Here's how the part is built. I have some questions about the finished solid (model axes, mm). A direction names the side the tool comes from. Round coordinates to 2 decimals unless told otherwise and drop trailing zeros. Loops run counter-clockwise (first coordinate to the right, second up) from the corner with the lowest first, then second, coordinate; pieces in that order, holes last. Notation, with made-up numbers: M 54,53.5 L 88,53.5 A25 ccw 88,80.5 Z; hole C -30,88.5 d11. An arc over 180 degrees is marked long. Answer as a JSON object with one key per item and string values.
Autodesk Inventor part; units mm, degrees
ref_plane "YZ Plane" through (0, 0, 0) normal (1, 0, 0) x (0, 1, 0)
ref_plane "XZ Plane" through (0, 0, 0) normal (0, 1, 0) x (-1, 0, 0)
ref_plane "XY Plane" through (0, 0, 0) normal (0, 0, 1) x (1, 0, 0)
sketch "Sketch1" plane through (0, 0, 0) normal (0, 0, 1) x (1, 0, 0)
  circle A0 centre (0, 0) radius 28 construction
  line L0 (75, -135) -> (-75, -135) construction
  line L1 (-75, -135) -> (-75, 65) construction
  line L2 (-75, 65) -> (75, 65) construction
  line L3 (75, 65) -> (75, -135) construction
  line L4 (75, -135) -> (-75, 65) construction
  line L5 (-75, -135) -> (75, 65) construction
  circle A1 centre (0, 0) radius 20
  circle A2 centre (-38.0423, -27.6393) radius 20
  circle A3 centre (-23.5114, -72.3607) radius 20
  circle A4 centre (23.5114, -72.3607) radius 20
  circle A5 centre (38.0423, -27.6393) radius 20
  circle A6 centre (0, -40) radius 62.5
  circle A7 centre (0, -40) radius 1.5
  circle A8 centre (0, -40) radius 4.05
  circle A9 centre (38.0423, -27.6393) radius 22.5 construction
  circle A10 centre (0, 0) radius 22.5 construction
  circle A11 centre (-38.0423, -27.6393) radius 22.5 construction
  circle A12 centre (-23.5114, -72.3607) radius 22.5 construction
  circle A13 centre (23.5114, -72.3607) radius 22.5 construction
  point P0 (0, -35)
  point P1 (0, -32)
  dimension "d0" = 56
  dimension "d1" = 150
  dimension "d2" = 200
  dimension "d3" = 135
  dimension "d4" = 40
  dimension "d7" = 360
  dimension "d9" = 40
  dimension "d10" = 125
  dimension "d11" = 3
  dimension "d12" = 8.1
  dimension "d17" = 45
  dimension "d20" = 360
  dimension "d22" = 8
extrude "Extrusion1" add sketch "Sketch1" along normal blind 10 contours A6
extrude "Extrusion2" add sketch "Sketch1" along normal blind 7 contours A8
hole "Hole1" at (0, -40, 0) at (0, -32, 0) direction (0, 0, 1) diameter 2 end through all
properties part number "FilterWheel-M40-5pos"
Item 1: For faces 1 (the face through (0, -42, 7)), 2 (the face through (20.91, -92.19, 4.93)), which set-ups out of +Z, -Z, +X, -X, +Y, -Y let a thin tool reach every point of the face, with its end or its side?
Solution:
{"face 1": "+Z", "face 2": "+Z, -Z"}
Item 2: If I drill on L1, parallel to Y at x = 0, z = 4.75; L2, parallel to Y at x = 0, z = 7.25; L3, parallel to Y at x = 36.5, z = 6.75, over which ranges is the centre line in solid material (lowest first)? Write a range as from..to.
Solution:
{"L1": "y = -102.5..-41.5, -38.5..-33, -31..-20, 20..22.5", "L2": "y = -102.5..-44.05, -35.95..-33, -31..-20, 20..22.5", "L3": "y = -90.73..-87.57, -57.15..-47.58, -7.7..10.73"}
Item 3: I want a section at A-A on x = 12. List the corners of the cut face in (y, z) for me.
Solution:
{"outline": "M -101.34,0 L -88.72,0 L -88.72,10 L -101.34,10 Z; M -56.01,0 L -16,0 L -16,10 L -56.01,10 Z; M 16,0 L 21.34,0 L 21.34,10 L 16,10 Z"}
Item 4: I want a section at D-D on z = 2. List the corners of the cut face in (x, y) for me.
Solution:
{"outline": "C 0,-40 d125; hole C -38.04,-27.64 d40; hole C -23.51,-72.36 d40; hole C 0,0 d40; hole C 0,-40 d3; hole C 0,-32 d2; hole C 23.51,-72.36 d40; hole C 38.04,-27.64 d40"}
Item 5: We'd pull the mould along X, two halves only. Please class faces 3 (the face through (-1, -53, 10)), 4 (the face through (-0.325, -38.536, 3.451)), 5 (the face through (-62.44, -42.75, 4.93)): +X half, -X half, draft (parallel to the pull), parting line (faces both ways), or undercut.
Solution:
{"face 3": "draft", "face 4": "undercut", "face 5": "parting line"}
Item 6: I want a section at C-C on y = -40. List the corners of the cut face in (x, z) for me.
Solution:
{"outline": "M -62.5,0 L -53.77,0 L -53.77,10 L -62.5,10 Z; M -22.32,0 L -1.5,0 L -1.5,7 L -4.05,7 L -4.05,10 L -22.32,10 Z; M 1.5,0 L 22.32,0 L 22.32,10 L 4.05,10 L 4.05,7 L 1.5,7 Z; M 53.77,0 L 62.5,0 L 62.5,10 L 53.77,10 Z"}
Item 7: I want a section at B-B on y = -54.5. List the corners of the cut face in (x, z) for me.
Solution:
{"outline": "M -60.79,0 L -32.51,0 L -32.51,10 L -60.79,10 Z; M -14.51,0 L 14.51,0 L 14.51,10 L -14.51,10 Z; M 32.51,0 L 60.79,0 L 60.79,10 L 32.51,10 Z"}
Item 8: For P1, Ø6, axis at x = 18, z = 5, coming from the +Y side; P2, Ø4, axis at x = -1.5, y = -41, coming from the +Z side; P3, Ø1.5, axis at x = 18, z = 4.5, coming from the -Y side, each with a flat end and sliding along its axis, tell me the tip position at first contact or that it passes through.
Solution:
{"P1": "stops at y = 20.67", "P2": "stops at z = 7", "P3": "stops at y = -100.07"}
